Work out the finished part from the listing and answer in its coordinate system (mm). A direction names the side the tool comes from. Give positions to 0.01 mm unless a question says otherwise; leave off trailing zeros. Write each loop counter-clockwise with the first axis right and the second up, starting at its lowest first coordinate (ties: lowest second). Pieces come first, ordered by that corner, then holes.
1) A tool of negligible diameter and unlimited length cuts with its end or side. For faces 1 (the face through (8.52, 10.34, -66.32)), 2 (the face through (41.61, 10.02, -10.99)), 3 (the face through (11, 8.859, -10)), 4 (the face through (63.048, -10, 42)), 5 (the face through (23.77, 17, 42)), from which of +Z, -Z, +X, -X, +Y, -Y can it reach the whole face along a straight path? Write none if from no direction.
2) Given pin 1 Ø6 at (x, y) = (-15, 6.5) entering from -Z; pin 2 Ø5 at (x, y) = (-21, -12) entering from +Z; pin 3 Ø6 at (x, z) = (42, 16) entering from +Y; pin 4 Ø8 at (x, y) = (14.5, 6.5) entering from +Z, each flat-ended and moving along its own axis, determine where each tip first touches the part or whether it passes through.
3) Find section C-C (z = 52). Determine the outline of the cut face in (x, y).
4) Straight lines are drawn through the part: probe 1 along Y at (x, z) = (-7.5, -69); probe 2 along Y at (x, z) = (15.5, 53); probe 3 along Y at (x, z) = (-33, -78). For each, find the intervals that lie inside material, in ascending order.
5) Find section D-D (y = 14). Count the separate pieces of the cut face and the enclosed holes in it, plus the area to 3 significant figures.
6) Find section B-B (x = -26). Determine the outline of the cut face in (y, z).
7) Find section A-A (y = -13.5). Determine the outline of the cut face in (x, z), plus the area to 3 significant figures.
8) Determine the mould class of faces 6 (the face through (63.376, -10.669, -16.733)), 7 (the face through (40.539, 10, 42)), 8 (the face through (28, -10.2, -77.6)) for opening direction Z: pulls with the +Z half, pulls with the -Z half, needs draft (parallel to the pull), parting line crosses it, or undercut.
```python
from build123d import *

# Parameters (mm, degrees)
F1_ANGLE = 30
F2_DEPTH = 84.6318360418
F3_DEPTH = 107.8587528318
F4_T     = -2.5


with BuildPart() as f1:
    # F0 (on Top) → F1 (revolve)
    with BuildSketch(Plane.XY):
        Polygon((40.5386388302, 0), (0, 0), (0, -32.6061099768), (65.5476081002, -32.6061099768), (65.5476081002, 10.6613785028), (56.5390067924, 34.8190441728), (14.7391783822, 34.0979024768), (12.93744918, 8.8585615158), (26.2701737512, 8.8585615158), (26.2701737512, 20.3965455294), (40.5386388302, 20.3965455294), align=None)
    revolve(axis=Axis((0, 33.5853546858, 0), (0, 1, 0)), revolution_arc=F1_ANGLE)

    # F2 (add): a face of the model
    f2_faces = [f1.faces().sort_by_distance(p)[0] for p in [
        (35.8528851523, -3.0790957236, 0),
    ]]
    extrude(f2_faces, amount=F2_DEPTH)

    # F3 (add): a face of the model
    f3_faces = [f1.faces().sort_by_distance(p)[0] for p in [
        (31.0495093409, -3.0790957236, -17.9264425762),
    ]]
    extrude(f3_faces, amount=F3_DEPTH)

    # F4
    f4_openings = [f1.faces().sort_by_distance(p)[0] for p in [
        (3.899671, 34.458473, -64.523756),
        (34.42472, 34.458473, -9.224076),
        (35.639093, 34.458473, 42.315918),
        (35.852885, -3.079096, 84.631836),
        (-22.879867, -3.079096, -111.334863),
    ]]
    offset(amount=F4_T, openings=f4_openings, kind=Kind.INTERSECTION)


solid = f1.part
```
Results:
1. face 1: none
1. face 2: +Y
1. face 3: +Z, -X
1. face 4: +Z
1. face 5: +Z, +Y
2. pin 1: stops at z = -114.93
2. pin 2: stops at z = -32.04
2. pin 3: stops at y = 22.9
2. pin 4: stops at z = 84.63
3. outline: (0, -32.61) - (65.55, -32.61) - (65.55, 10.66) - (56.54, 34.82) - (53.89, 34.77) - (63.05, 10.21) - (63.05, -30.11) - (2.5, -30.11) - (2.5, -2.5) - (43.04, -2.5) - (43.04, 22.9) - (23.77, 22.9) - (23.77, 11.36) - (15.62, 11.36) - (17.25, 34.14) - (14.74, 34.1) - (12.94, 8.86) - (26.27, 8.86) - (26.27, 20.4) - (40.54, 20.4) - (40.54, 0) - (0, 0) - close
4. probe 1: y = -32.61 to -30.11, -2.5 to 0, 20.4 to 22.9
4. probe 2: y = -32.61 to -30.11, -2.5 to 0, 8.86 to 34.11
4. probe 3: y = -32.61 to -30.11, -2.5 to 0
5. separate pieces: 4
5. enclosed holes: 0
5. area: 2,150 mm2
6. outline: (-32.61, -109.53) - (-30.11, -109.53) - (-30.11, -50.03) - (-2.5, -50.03) - (-2.5, -109.53) - (0, -109.53) - (0, -45.03) - (-32.61, -45.03) - close; (8.86, -97.57) - (20.4, -97.57) - (20.4, -109.53) - (22.9, -109.53) - (22.9, -92.57) - (11.36, -92.57) - (11.36, -76.28) - (34.14, -79.53) - (34.1, -74.51) - (8.86, -70.91) - close
7. outline: (-53.93, -93.41) - (-51.76, -94.66) - (2.5, -0.67) - (2.5, 84.63) - (0, 84.63) - (0, 0) - close; (0.67, -124.93) - (2.84, -126.18) - (56.77, -32.77) arc R65.55 ccw to (65.55, 0) - (65.55, 84.63) - (63.05, 84.63) - (63.05, 0) arc R63.05 cw to (54.6, -31.52) - close
7. area: 1,050 mm2
8. face 6: pulls with the -Z half
8. face 7: needs draft
8. face 8: undercut
